```python
from build123d import *

# Parameters (mm, degrees)
SKETCH1_W               = 63.5
SKETCH1_H               = 134.62
SKETCH1_R               = 6.35
BOSS_EXTRUDE1_DEPTH     = 12.7
SKETCH2_W               = 63.5
SKETCH2_H               = 33.02
CUT_EXTRUDE1_DEPTH      = 76.498268854
F_1_4_CLEARANCE_HOLE1_D = 6.7564


with BuildPart() as part:
    # Sketch1 → Boss-Extrude1 (new body)
    with BuildSketch(Plane.XY):
        Rectangle(SKETCH1_W, SKETCH1_H)
        with Locations((-9.26084, 0)):
            Circle(SKETCH1_R, mode=Mode.SUBTRACT)
        with Locations((9.26084, 0)):
            Circle(SKETCH1_R, mode=Mode.SUBTRACT)
    extrude(amount=BOSS_EXTRUDE1_DEPTH)

    # Sketch2 → Cut-Extrude1 (cut, through all)
    with BuildSketch(Plane.XY.offset(12.7)):
        with Locations((0, 50.8)):
            Rectangle(SKETCH2_W, SKETCH2_H)
    extrude(amount=-CUT_EXTRUDE1_DEPTH, mode=Mode.SUBTRACT)

    # 1/4 Clearance Hole1 (through all)
    with Locations(Plane.XY.offset(12.7)):
        with Locations((-21.59, 24.13)):
            f_1_4_clearance_hole1 = Hole(F_1_4_CLEARANCE_HOLE1_D / 2)

    # Mirror1: 1/4 Clearance Hole1 across plane
    add(f_1_4_clearance_hole1.mirror(Plane(origin=(0, 0, 0), x_dir=(0, 0, 1), z_dir=(1, 0, 0))), mode=Mode.SUBTRACT)

    # Sketch8 → #10-32 Tapped Hole1 (revolve, cut)
    with BuildSketch(Plane(origin=(-21.59, -67.31, 6.35), x_dir=(0, 0, -1), z_dir=(1, 0, 0))):
        Polygon((0, 0), (0, 26.613317848), (2.0193, 25.4), (2.0193, 0), align=None)
    f_10_32_tapped_hole1 = revolve(axis=Axis((-21.59, -73.66, 6.35), (0, 1, 0)), mode=Mode.SUBTRACT)

    # Mirror2: #10-32 Tapped Hole1 across plane
    add(f_10_32_tapped_hole1.mirror(Plane(origin=(0, 0, 0), x_dir=(0, 0, 1), z_dir=(1, 0, 0))), mode=Mode.SUBTRACT)


solid = part.part
```
The listing builds one solid part. Answer for the finished solid, in the listing's coordinates (mm). A direction names the side the tool comes from. Coordinates: 2 decimals unless noted, no trailing zeros. Loops run counter-clockwise (first coordinate to the right, second up) from the corner with the lowest first, then second, coordinate; pieces in that order, holes last. Notation, with made-up numbers: (-15, 39.25) -> (12, 39.25) arc R20 cw to (12, 48.25) -> close; hole circle Ø6 at (52, -32). An arc over 180 degrees is marked (long way). Return JSON: item names as keys, results as strings. Group by question number.
(1) Determine the mould class of faces 1 (the conical face through (21.94, -40.91, 6.4)), 2 (the flat face through (31.75, -17, 6)), 3 (the flat face through (0, -67.31, 6)) for opening direction X: released by +X, released by -X, zero draft, split by the parting line, or undercut.
(2) Which of the six approach directions +Z, -Z, +X, -X, +Y, -Y give full straight-line access (tool end or side, diameter ignored) to faces 4 (the cylindrical face through (20.86, 20.83, 6.26)), 5 (the cylindrical face through (-19.62, -54.79, 6.79))?
(3) A cutting plane is placed at A-A on y = 24.13. Write down the section's boundary in (x, z), and give its area (3 significant figures).
(4) Given pin 1 Ø10 at (x, y) = (-9.26, 0) entering from -Z, flat-ended and moving along its own axis, determine where the tip first touches the part or whether it passes through.
(5) A cutting plane is placed at D-D on x = 6.5. Write down the section's boundary in (y, z).
(6) Find the intervals of material crossed by probe 1 along X at (y, z) = (-53, 6.35); probe 2 along X at (y, z) = (26, 2.5); probe 3 along Y at (x, z) = (19.5, 5), in increasing order. Write a range as from..to.
(7) A cutting plane is placed at C-C on y = -57.5. Write down the section's boundary in (x, z), and give its area (3 significant figures).
(8) A cutting plane is placed at B-B on z = 10. Write down the section's boundary in (x, y).
The answers:
{
 "1": {"face 1": "undercut", "face 2": "released by +X", "face 3": "zero draft"},
 "2": {"face 4": "+Z, -Z", "face 5": "-Y"},
 "3": {"outline": "(-31.75, 0) -> (-24.97, 0) -> (-24.97, 12.7) -> (-31.75, 12.7) -> close; (-18.21, 0) -> (18.21, 0) -> (18.21, 12.7) -> (-18.21, 12.7) -> close; (24.97, 0) -> (31.75, 0) -> (31.75, 12.7) -> (24.97, 12.7) -> close", "area": "635 mm^2"},
 "4": {"pin 1": "passes through"},
 "5": {"outline": "(-67.31, 0) -> (-5.72, 0) -> (-5.72, 12.7) -> (-67.31, 12.7) -> close; (5.72, 0) -> (34.29, 0) -> (34.29, 12.7) -> (5.72, 12.7) -> close"},
 "6": {"probe 1": "x = -31.75..-23.61, -19.57..19.57, 23.61..31.75", "probe 2": "x = -31.75..-24.4, -18.78..18.78, 24.4..31.75", "probe 3": "y = -67.31..21.48, 26.78..34.29"},
 "7": {"outline": "(-31.75, 0) -> (31.75, 0) -> (31.75, 12.7) -> (-31.75, 12.7) -> close; hole circle Ø4.04 at (-21.59, 6.35); hole circle Ø4.04 at (21.59, 6.35)", "area": "781 mm^2"},
 "8": {"outline": "(-31.75, -67.31) -> (31.75, -67.31) -> (31.75, 34.29) -> (-31.75, 34.29) -> close; hole circle Ø6.76 at (-21.59, 24.13); hole circle Ø12.7 at (-9.26, 0); hole circle Ø12.7 at (9.26, 0); hole circle Ø6.76 at (21.59, 24.13)"}
}
